Work out the finished part from the listing and answer in its coordinate system (mm). Coordinates: 2 decimals unless noted, no trailing zeros. Write each loop counter-clockwise with the first axis right and the second up, starting at its lowest first coordinate (ties: lowest second). Pieces come first, ordered by that corner, then holes. Notation, with made-up numbers: (-14, 40) - (3, 40) arc R8 cw to (3, 46) - close; hole circle Ø3 at (-20.75, 55). An arc over 180 degrees is marked (long way). Use a Markdown table: item, result. Add a question column.
(1) Find the intervals of material crossed by line 1 (Y direction, x = 0, z = 104.35); line 2 (Z direction, x = 0, y = 0.5); line 3 (Y direction, x = 5.25, z = 98), in increasing order. Write a range as from..to.
(2) Given pin 1 Ø4 at (y, z) = (-3, 95) entering from -X; pin 2 Ø3 at (x, y) = (0, 0) entering from +Z; pin 3 Ø5 at (y, z) = (3, 77.5) entering from +X, each flat-ended and moving along its own axis, determine where each tip first touches the part or whether it passes through.
(3) The part is cut by section D-D, the plane x = -3. Give the vertices of the cut face in (y, z).
(4) The part is cut by section B-B, the plane y = -0.75. Give the vertices of the cut face in (x, z).
(5) The part is cut by section A-A, the plane x = -1.5. Give the vertices of the cut face in (y, z), then the cut area to 3 significant figures.
(6) The part is cut by section C-C, the plane z = 80. Give the vertices of the cut face in (x, y), then the cut area to 3 significant figures.
from build123d import *

# Parameters (mm, degrees)
IZIM1_R                     = 30
Y_KSEKLIK_EKSTR_ZYON1_DEPTH = 175
IZIM5_R                     = 10
KES_EKSTR_ZYON1_DEPTH       = 5
L_EK1_SCALE                 = 0.2


with BuildPart() as part:
    # Çizim1 → Yükseklik-Ekstrüzyon1 (new body)
    with BuildSketch(Plane.XY):
        Circle(IZIM1_R)
    extrude(amount=Y_KSEKLIK_EKSTR_ZYON1_DEPTH)

    # Çizim5 → Kes-Ekstrüzyon1 (cut)
    with BuildSketch(Plane.XY.offset(175)):
        Circle(IZIM5_R)
    extrude(amount=-KES_EKSTR_ZYON1_DEPTH, mode=Mode.SUBTRACT)


with BuildPart() as part_1:
    # Ölçek1: scaled about (0, 0, 87.229299363)
    add(part.part.scale(L_EK1_SCALE).moved(Location((0, 0, 69.78343949))))


solid = part_1.part
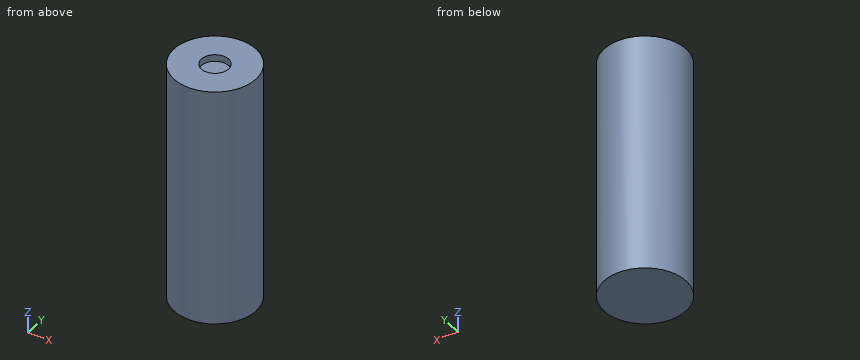
Model answer:
| question | item | result |
|---|---|---|
| 1 | line 1 | -6..-2, 2..6 |
| 1 | line 2 | 69.78..103.78 |
| 1 | line 3 | -2.9..2.9 |
| 2 | pin 1 | x = -5.92 |
| 2 | pin 2 | z = 103.78 |
| 2 | pin 3 | x = 5.98 |
| 3 | outline | (-5.2, 69.78) - (5.2, 69.78) - (5.2, 104.78) - (-5.2, 104.78) - close |
| 4 | outline | (-5.95, 69.78) - (5.95, 69.78) - (5.95, 104.78) - (1.85, 104.78) - (1.85, 103.78) - (-1.85, 103.78) - (-1.85, 104.78) - (-5.95, 104.78) - close |
| 5 | outline | (-5.81, 69.78) - (5.81, 69.78) - (5.81, 104.78) - (1.32, 104.78) - (1.32, 103.78) - (-1.32, 103.78) - (-1.32, 104.78) - (-5.81, 104.78) - close |
| 5 | area | 404 mm^2 |
| 6 | outline | circle Ø12 at (0, 0) |
| 6 | area | 113 mm^2 |
